```python
from build123d import *

# Parameters (mm, degrees)
BOSS_EXTRUDE1_DEPTH = 80
SKETCH2_W           = 36.5
SKETCH2_H           = 80
CUT_EXTRUDE1_DEPTH  = 9
SKETCH3_W           = 50
SKETCH3_H           = 80
SKETCH3_W_2         = 25
SKETCH3_H_2         = 72
BOSS_EXTRUDE2_DEPTH = 2


with BuildPart() as part:
    # Sketch1 → Boss-Extrude1 (new body)
    with BuildSketch(Plane(origin=(0, 0, 0), x_dir=(1, 0, 0), z_dir=(0, 1, 0))):
        Polygon((89.086021447, 0.382365888), (91.207341791, 2.503686231), (55.852002731, 37.859025291), (53.730682388, 35.737704947), (53.377128997, 35.487704947), (45.806568717, 35.487704947), (88.836021447, -7.499362096), (88.836021447, 0.028812497), align=None)
    extrude(amount=BOSS_EXTRUDE1_DEPTH)

    # Sketch2 → Cut-Extrude1 (cut)
    with BuildSketch(Plane(origin=(46.855514011, 0, -46.855514011), x_dir=(-0.707106781, 0, -0.707106781), z_dir=(0.707106781, 0, -0.707106781))):
        with Locations((-37.722956362, 40)):
            Rectangle(SKETCH2_W, SKETCH2_H)
    extrude(amount=-CUT_EXTRUDE1_DEPTH, mode=Mode.SUBTRACT)

    # Sketch3 → Boss-Extrude2 (add)
    with BuildSketch(Plane(origin=(46.855514011, 0, -46.855514011), x_dir=(-0.707106781, 0, -0.707106781), z_dir=(0.707106781, 0, -0.707106781))):
        with Locations((-37.722956362, 40)):
            Rectangle(SKETCH3_W, SKETCH3_H)
        with Locations((-37.722956362, 40)):
            Rectangle(SKETCH3_W_2, SKETCH3_H_2, mode=Mode.SUBTRACT)
    extrude(amount=-BOSS_EXTRUDE2_DEPTH)


solid = part.part
```
Build history of the part. All positions in model axes, mm. A direction names the side the tool comes from. Coordinates: 2 decimals unless noted, no trailing zeros. Order: outer loops, then holes, each group sorted by start corner. A loop starts at its lowest first (then second) coordinate and runs counter-clockwise, first axis right, second up.
Item 1: Saw through at A-A on y = 60.5. List the corners of the cut face in (x, z), then the cut area to 3 significant figures.
Filled in:
outline: (45.81, -35.49) - (53.38, -35.49) - (53.73, -35.74) - (55.85, -37.86) - (64.69, -29.02) - (63.28, -27.61) - (59.21, -31.67) - (54.42, -26.88) - close; (80.24, -1.09) - (85.02, -5.86) - (80.95, -9.93) - (82.37, -11.34) - (91.21, -2.5) - (89.09, -0.38) - (88.84, -0.03) - (88.84, 7.5) - close
area: 171 mm2
Item 2: Saw through at D-D on x = 87.5. List the corners of the cut face in (y, z).
Filled in:
outline: (0, -6.21) - (80, -6.21) - (80, 6.16) - (0, 6.16) - close
Item 3: Saw through at C-C on x = 76. List the corners of the cut face in (y, z).
Filled in:
outline: (0, -17.71) - (4, -17.71) - (4, -14.88) - (0, -14.88) - close; (76, -17.71) - (80, -17.71) - (80, -14.88) - (76, -14.88) - close
Item 4: Drop flat-ended pins along their axis: pin 1 Ø3 at (x, y) = (57, 46.5) entering from -Z; pin 2 Ø10 at (x, z) = (67, -30.5) entering from -Y; pin 3 Ø12 at (y, z) = (18.5, -28) entering from -X; pin 4 Ø6 at (x, y) = (64, 8.5) entering from -Z. Give the stop position or say it passes through.
Filled in:
pin 1: stops at z = -37.86
pin 2: stops at y = 0
pin 3: stops at x = 47.3
pin 4: stops at z = -32.71
Item 5: Tool access for faces 1 (the flat face through (56.85, 39.44, -29.31)), 2 (the flat face through (88.836, 39, 4)), 3 (the flat face through (82.665, 39.44, -3.507)), 4 (the flat face through (50, 39, -35.488)): list every direction of +Z, -Z, +X, -X, +Y, -Y with a clear straight run to the whole face (end or side of a thin tool).
Filled in:
face 1: +Z, +Y, -Y
face 2: +Z, +X, +Y, -Y
face 3: -X, +Y, -Y
face 4: -Z, -X, +Y, -Y
Item 6: Saw through at B-B on z = -30.5. List the corners of the cut face in (x, y).
Filled in:
outline: (50.8, 0) - (58.04, 0) - (58.04, 80) - (50.8, 80) - close; (60.38, 0) - (63.21, 0) - (63.21, 80) - (60.38, 80) - close
Item 7: Drill centre lines: L1, parallel to Z at x = 89, y = 26.5; L2, parallel to X at y = 6.5, z = 1; L3, parallel to Z at x = 62, y = 46.5. Where is each one in solid material? Low to high.
Filled in:
L1: z = -4.71 to -0.26
L2: x = 82.33 to 88.84
L3: z = -31.71 to -28.88
Item 8: Mould opens along X. For faces 5 (the flat face through (73, 0, -19)), 6 (the flat face through (84.48, 39.44, 3.15)), 7 (the flat face through (90.132, 39.44, -1.428)), 8 (the flat face through (81.73, 37.22, -9.15)) say: released by +X, released by -X, zero draft, split by the parting line, or undercut.
Filled in:
face 5: zero draft
face 6: released by -X
face 7: released by +X
face 8: undercut
